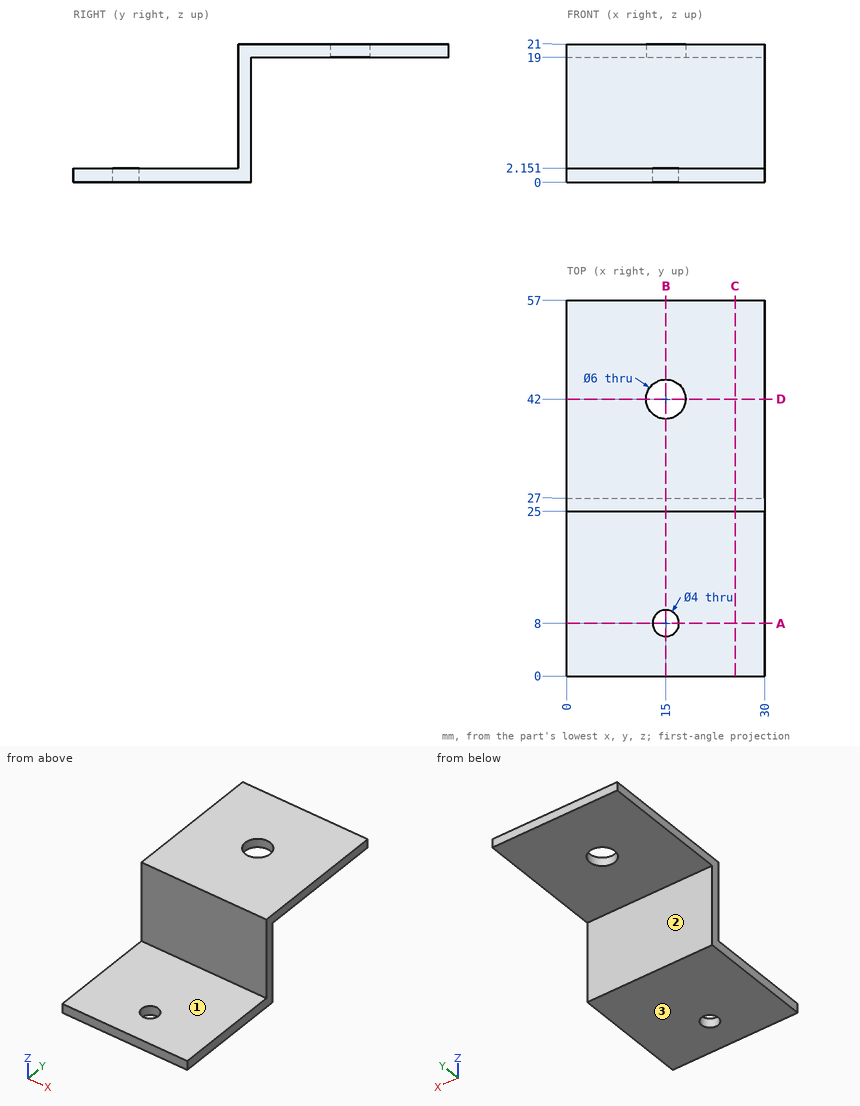
Geometry check sheet. Reference: drawing and pictorial views, mm from the part's lowest x, y, z. A direction names the side the tool comes from. Give positions to 0.01 mm unless a question says otherwise; leave off trailing zeros. Order: outer loops, then holes, each group sorted by start corner. A loop starts at its lowest first (then second) coordinate and runs counter-clockwise, first axis right, second up. Notation, with made-up numbers: M 87,75 L 91,75 A24 cw 91,95 Z; hole C -13.75,-32.5 d6. An arc over 180 degrees is marked long. Return JSON: item names as keys, results as strings. Group by question number.
1) Section check B-B on x = 15. Record the cut outline in (y, z).
2) Section check A-A on y = 8. Record the cut outline in (x, z).
3) Access from +Z, -Z, +X, -X, +Y, -Y to the whole of each face (thin tool, end or side, straight path). Record for the marked faces 1, 2 and 3.
4) Scan lines: line 1 (Y direction, x = 15, z = 20.15); line 2 (X direction, y = 42, z = 20.25); line 3 (Z direction, x = 24.75, y = 13). Record each from-to range of solid material in increasing order.
5) Section check D-D on y = 42. Record the cut outline in (x, z), and give its area (3 significant figures).
6) Go/stop test with flat-tipped pins: pin 1 Ø4 at (x, z) = (16.5, 9.5) entering from -Y; pin 2 Ø1.5 at (x, z) = (22.5, 7.5) entering from +Y; pin 3 Ø5 at (y, z) = (23, 16) entering from -X. Record where each tip stops, or that it passes through.
7) Section check C-C on x = 25.5. Record the cut outline in (y, z).
Answer block:
{
 "1": {"outline": "M 0,0 L 6,0 L 6,2.15 L 0,2.15 Z; M 10,0 L 27,0 L 27,19 L 39,19 L 39,21 L 25,21 L 25,2.15 L 10,2.15 Z; M 45,19 L 57,19 L 57,21 L 45,21 Z"},
 "2": {"outline": "M 0,0 L 13,0 L 13,2.15 L 0,2.15 Z; M 17,0 L 30,0 L 30,2.15 L 17,2.15 Z"},
 "3": {"face 1": "+Z, +X, -X, -Y", "face 2": "-Z, +X, -X, +Y", "face 3": "-Z, +X, -X, +Y, -Y"},
 "4": {"line 1": "y = 25 to 39, 45 to 57", "line 2": "x = 0 to 12, 18 to 30", "line 3": "z = 0 to 2.15"},
 "5": {"outline": "M 0,19 L 12,19 L 12,21 L 0,21 Z; M 18,19 L 30,19 L 30,21 L 18,21 Z", "area": "48.0 mm^2"},
 "6": {"pin 1": "stops at y = 25", "pin 2": "stops at y = 27", "pin 3": "stops at x = 0"},
 "7": {"outline": "M 0,0 L 27,0 L 27,19 L 57,19 L 57,21 L 25,21 L 25,2.15 L 0,2.15 Z"}
}
